Source: CAD feature listing. Evaluate the final solid. Frame: model axes, mm. Round coordinates to 2 decimals unless told otherwise and drop trailing zeros. Order: outer loops, then holes, each group sorted by start corner. A loop starts at its lowest first (then second) coordinate and runs counter-clockwise, first axis right, second up. Notation, with made-up numbers: M -28.75,23.5 L 24.25,23.5 A26 cw 24.25,59.5 Z; hole C 2.5,89 d4. An arc over 180 degrees is marked long. Use one line per item in the form item = value. Start each with the question number.
Q1. Material intervals for probe 1 along X at (y, z) = (-18.5, 43); probe 2 along X at (y, z) = (-21.5, 38); probe 3 along X at (y, z) = (-12, 32.5), sorted ascending.
Q2. Contact query for flat-ended pins moving along their axis: pin 1 (1.5 mm diameter, centred on x = -21.5, y = -21.5, fed in from +Z); pin 2 (1 mm diameter, centred on x = 7, y = -17, fed in from -Z). Output: stop coordinate, or through.
Q3. Section B-B (x = -45). Return the cut outline in (y, z).
from build123d import *

# Parameters (mm, degrees)
F0_R     = 5.7858017693
F0_R_2   = 12.2144234622
F1_DEPTH = 25.4
F2_R     = 6.35
F3_DEPTH = 25.4
F4_DEPTH = 25.4
F5_R     = 11.3360487182
F5_R_2   = 5.404630024
F6_DEPTH = 143.764


with BuildPart() as f1:
    # F0 (on Front) → F1 (new body)
    with BuildSketch(Plane.XZ):
        with BuildLine():
            Line((12.9150417295, 54.2136049138), (-58.6621068715, 60.7312914672))
            ThreePointArc((-58.6621068715, 60.7312914672), (-47.6420330376, 53.6105540281), (-43.3609664676, 41.2081591785))
            ThreePointArc((-43.3609664676, 41.2081591785), (-47.549687182, 28.9245030523), (-58.370527571, 21.7590999007))
            Line((-58.370527571, 21.7590999007), (12.9064416896, 28.2019332059))
            ThreePointArc((12.9064416896, 28.2019332059), (-1.3284624626, 41.2124768589), (12.9150417295, 54.2136049138))
        make_face()
        with BuildLine():
            ThreePointArc((24.7900415902, 41.2081591785), (21.374686899, 50.0137999909), (12.9150417295, 54.2136049138))
            ThreePointArc((12.9150417295, 54.2136049138), (-1.3284624626, 41.2124768589), (12.9064416896, 28.2019332059))
            ThreePointArc((12.9064416896, 28.2019332059), (21.3717750304, 32.3993303595), (24.7900415902, 41.2081591785))
        make_face()
        with Locations((11.7307892069, 41.2081591785)):
            Circle(F0_R, mode=Mode.SUBTRACT)
        with BuildLine():
            ThreePointArc((-58.6621068715, 60.7312914672), (-61.6433409645, 61.2309324181), (-64.6657877732, 61.2779758637))
            Line((-64.6657877732, 61.2779758637), (-58.6621068715, 60.7312914672))
        make_face()
        with BuildLine():
            Line((-58.370527571, 21.7590999007), (-64.9924645965, 21.1605329743))
            ThreePointArc((-64.9924645965, 21.1605329743), (-61.6565813141, 21.1841847102), (-58.370527571, 21.7590999007))
        make_face()
        with Locations((11.7307892069, 41.2081591785)):
            Circle(F0_R)
        with BuildLine():
            Line((-58.6621068715, 60.7312914672), (-64.6657877732, 61.2779758637))
            ThreePointArc((-64.6657877732, 61.2779758637), (-83.5715244216, 41.3718739948), (-64.9924645965, 21.1605329743))
            Line((-64.9924645965, 21.1605329743), (-58.370527571, 21.7590999007))
            ThreePointArc((-58.370527571, 21.7590999007), (-47.549687182, 28.9245030523), (-43.3609664676, 41.2081591785))
            ThreePointArc((-43.3609664676, 41.2081591785), (-47.6420330376, 53.6105540281), (-58.6621068715, 60.7312914672))
        make_face()
        with Locations((-63.466578722, 41.2081591785)):
            Circle(F0_R_2, mode=Mode.SUBTRACT)
        with Locations((-63.466578722, 41.2081591785)):
            Circle(F0_R_2)
    extrude(amount=F1_DEPTH)

    # F4 (add): a face of the model
    f4_faces = [f1.faces().sort_by_distance(p)[0] for p in [
        (-33.0156051896, -25.4, 41.2168506506),
    ]]
    extrude(f4_faces, amount=F4_DEPTH)

    # F5 (on face) → F6 (cut)
    with BuildSketch(Plane.XZ.offset(50.8)):
        with Locations((-63.466578722, 41.2081591785)):
            Circle(F5_R)
        with Locations((11.7307892069, 41.2081591785)):
            Circle(F5_R_2)
    extrude(amount=-F6_DEPTH, mode=Mode.SUBTRACT)


with BuildPart() as f3:
    # F2 (on Front) → F3 (new body)
    with BuildSketch(Plane.XZ):
        with Locations((-100.2000197768, -20.0504176319)):
            Circle(F2_R)
    extrude(amount=F3_DEPTH)


solid = f1.part
Results list:
q1.probe_1 = -83.49 to -74.66, -52.27 to 6.63, 16.83 to 24.67
q1.probe_2 = -83.31 to -74.34, -52.59 to 7.38, 16.08 to 24.39
q1.probe_3 = -81.59 to -70.72, -56.21 to 21.46
q2.pin_1 = 57.42
q2.pin_2 = 27.62
q3.outline = M -50.8,22.97 L 0,22.97 L 0,59.49 L -50.8,59.49 Z
